Could you check a few things on this model? Use its own coordinates, in mm. A direction names the side the tool comes from. Give positions to 0.01 mm unless a question says otherwise; leave off trailing zeros. Loops run counter-clockwise (first coordinate to the right, second up) from the corner with the lowest first, then second, coordinate; pieces in that order, holes last. Notation, with made-up numbers: (11, 20) -> (29, 20) arc R19 ccw to (29, 41) -> close; hole circle Ø8 at (69.25, -37). An arc over 180 degrees is marked (long way). Write item = value, one per line. Start each with the question number.
1) I'm going to push a flat-ended pin straight in: pin 1 Ø13 at (x, z) = (-31, -98) entering from +Y. Where does the tip first touch, or does it pass through?
2) I want a section at B-B (x = 23). Count the separate pieces of the cut face and the enclosed holes in it, and give its area (3 significant figures).
3) I need wall thicknesses on probe 1 along Z at (x, y) = (24.5, 9); probe 2 along X at (y, z) = (4, -111); probe 3 along Y at (x, z) = (35, 29). Which ranges of each line are inside material? Lowest first, please. Write a range as from..to.
4) On a 3-axis mill with a long thin cutter (end or side, diameter ignored), from which of +Z, -Z, +X, -X, +Y, -Y can I reach the whole of each face in a straight line? I mean faces 1 (the face through (-1, 3, 15)), 2 (the face through (-1, 0, 6)), 3 (the face through (-1, 10, 145)). Say none if no direction works.
5) I want a section at A-A (z = 21). List the corners of the cut face in (x, y) for me, and give its area (3 significant figures).
6) If we mould it in two halves opening along Z, with no side actions, what happens to faces 4 (the face through (-1, 7, 150)), 5 (the face through (-1, 3, 119)), 6 (the face through (77, 10, -37)), 7 (the face through (-1, 3, 67))? For each: +Z half, -Z half, draft (parallel to the pull), parting line (faces both ways), or undercut.
7) I want a section at C-C (z = 80.5). List the corners of the cut face in (x, y) for me, and give its area (3 significant figures).
from build123d import *

# Parameters (mm, degrees)
TRAY_W              = 160
TRAY_H              = 285
BOSS_EXTRUDE1_DEPTH = 5
BOSS_EXTRUDE2_DEPTH = 5
SKETCH3_W           = 160
SKETCH3_H           = 5
BOSS_EXTRUDE3_DEPTH = 10
SKETCH4_W           = 150
SKETCH4_H           = 10
CUT_EXTRUDE1_DEPTH  = 171.293863659


with BuildPart() as part:
    # Tray → Boss-Extrude1 (new body)
    with BuildSketch(Plane(origin=(0, 0, 0), x_dir=(1, 0, 0), z_dir=(0, 1, 0))):
        with Locations((0, -7.5)):
            Rectangle(TRAY_W, TRAY_H)
    extrude(amount=BOSS_EXTRUDE1_DEPTH)

    # tray frame → Boss-Extrude2 (add)
    with BuildSketch(Plane(origin=(0, 5, 0), x_dir=(1, 0, 0), z_dir=(0, 1, 0))):
        Polygon((-80, -145), (-75, -145), (-75, 130), (75, 130), (75, -145), (80, -145), (80, 135), (-80, 135), align=None)
    extrude(amount=BOSS_EXTRUDE2_DEPTH)

    # Sketch3 → Boss-Extrude3 (add)
    with BuildSketch(Plane(origin=(0, 5, 0), x_dir=(1, 0, 0), z_dir=(0, 1, 0))):
        with Locations((0, -147.5)):
            Rectangle(SKETCH3_W, SKETCH3_H)
    extrude(amount=BOSS_EXTRUDE3_DEPTH)

    # Sketch4 → Cut-Extrude1 (cut, through all)
    with BuildSketch(Plane(origin=(0, 5, 0), x_dir=(1, 0, 0), z_dir=(0, 1, 0))):
        with Locations((0, 110)):
            Rectangle(SKETCH4_W, SKETCH4_H)
        with Locations((0, 84)):
            Rectangle(SKETCH4_W, SKETCH4_H)
        with Locations((0, 32)):
            Rectangle(SKETCH4_W, SKETCH4_H)
        with Locations((0, 6)):
            Rectangle(SKETCH4_W, SKETCH4_H)
        with Locations((0, -20)):
            Rectangle(SKETCH4_W, SKETCH4_H)
        with Locations((0, -46)):
            Rectangle(SKETCH4_W, SKETCH4_H)
        with Locations((0, -72)):
            Rectangle(SKETCH4_W, SKETCH4_H)
        with Locations((0, -98)):
            Rectangle(SKETCH4_W, SKETCH4_H)
        with Locations((0, -124)):
            Rectangle(SKETCH4_W, SKETCH4_H)
        with Locations((0, 58)):
            Rectangle(SKETCH4_W, SKETCH4_H)
    extrude(amount=-CUT_EXTRUDE1_DEPTH, mode=Mode.SUBTRACT)


solid = part.part
Answer list:
q1.pin_1 = 5
q2.separate_pieces = 11
q2.enclosed_holes = 0
q2.area = 1,000 mm^2
q3.probe_1 = -135..-130, 145..150
q3.probe_2 = -80..-75, 75..80
q3.probe_3 = 0..5
q4.face_1 = +Y, -Y
q4.face_2 = +Z, -Z, +X, -X, -Y
q4.face_3 = +Y
q5.outline = (-80, 0) -> (-75, 0) -> (-75, 10) -> (-80, 10) -> close; (75, 0) -> (80, 0) -> (80, 10) -> (75, 10) -> close
q5.area = 100 mm^2
q6.face_4 = +Z half
q6.face_5 = undercut
q6.face_6 = draft
q6.face_7 = undercut
q7.outline = (-80, 0) -> (80, 0) -> (80, 10) -> (75, 10) -> (75, 5) -> (-75, 5) -> (-75, 10) -> (-80, 10) -> close
q7.area = 850 mm^2
